from build123d import *

# Parameters (mm, degrees)
SKETCH_2_R      = 1.7
EXTRUDE_1_DEPTH = 3
EXTRUDE_2_DEPTH = 3.5
FILLET_5_R      = 1


with BuildPart() as part:
    # ｽｹｯﾁ2 → ﾎﾞｽ - 押し出し1 (new body)
    with BuildSketch(Plane(origin=(0, 0, 0), x_dir=(1, 0, 0), z_dir=(0, 1, 0))):
        with BuildLine():
            Line((85.95, 71.05), (89.45, 71.05))
            ThreePointArc((89.45, 71.05), (93.45, 67.05), (89.45, 63.05))
            Line((89.45, 63.05), (85.95, 63.05))
            Line((85.95, 63.05), (85.95, 8))
            Line((85.95, 8), (89.45, 8))
            ThreePointArc((89.45, 8), (93.45, 4), (89.45, 0))
            Line((89.45, 0), (85.95, 0))
            Line((85.95, 0), (0, 0))
            Line((0, 0), (-3.5, 0))
            ThreePointArc((-3.5, 0), (-7.5, 4), (-3.5, 8))
            Line((-3.5, 8), (0, 8))
            Line((0, 8), (0, 63.05))
            Line((0, 63.05), (-3.5, 63.05))
            ThreePointArc((-3.5, 63.05), (-7.5, 67.05), (-3.5, 71.05))
            Line((-3.5, 71.05), (0, 71.05))
            Line((0, 71.05), (85.95, 71.05))
        make_face()
        with Locations(Location((89.45, 67.05, 0), (0, 0, 270))):
            Circle(SKETCH_2_R, mode=Mode.SUBTRACT)
        with Locations(Location((89.45, 4, 0), (0, 0, 270))):
            Circle(SKETCH_2_R, mode=Mode.SUBTRACT)
        with Locations(Location((-3.5, 67.05, 0), (0, 0, 270))):
            Circle(SKETCH_2_R, mode=Mode.SUBTRACT)
        with Locations(Location((-3.5, 4, 0), (0, 0, 270))):
            Circle(SKETCH_2_R, mode=Mode.SUBTRACT)
    extrude(amount=EXTRUDE_1_DEPTH)

    # ｽｹｯﾁ3 → ﾎﾞｽ - 押し出し2 (add)
    with BuildSketch(Plane(origin=(0, 3, 0), x_dir=(1, 0, 0), z_dir=(0, 1, 0))):
        Polygon((68.9, 0), (70.5, 5.5), (70.5, 7.5), (67.5, 7.5), (67.5, 0), align=None)
        Polygon((67.5, 15.5), (70.5, 15.5), (70.5, 70.05), (82.95, 70.05), (82.95, 0), (85.95, 0), (85.95, 71.05), (67.5, 71.05), align=None)
        Polygon((45, 15.5), (48, 15.5), (48, 70.05), (60.45, 70.05), (60.45, 0), (63.45, 0), (63.45, 71.05), (45, 71.05), align=None)
        Polygon((46.4, 0), (48, 5.5), (48, 7.5), (45, 7.5), (45, 0), align=None)
        Polygon((22.5, 15.5), (25.5, 15.5), (25.5, 70.05), (37.95, 70.05), (37.95, 0), (40.95, 0), (40.95, 71.05), (22.5, 71.05), align=None)
        Polygon((23.9, 0), (25.5, 5.5), (25.5, 7.5), (22.5, 7.5), (22.5, 0), align=None)
        Polygon((0, 15.5), (3, 15.5), (3, 70.05), (15.45, 70.05), (15.45, 0), (18.45, 0), (18.45, 71.05), (0, 71.05), align=None)
        Polygon((1.4, 0), (3, 5.5), (3, 7.5), (0, 7.5), (0, 0), align=None)
    extrude(amount=EXTRUDE_2_DEPTH)

    # ﾌｨﾚｯﾄ5
    fillet_5_edges = [part.edges().sort_by_distance(p)[0] for p in [
        (85.95, 4.75, 0),
        (85.95, 4.75, -71.05),
        (45, 4.75, -71.05),
        (60.45, 4.75, 0),
        (63.45, 4.75, 0),
        (63.45, 4.75, -71.05),
        (22.5, 4.75, 0),
        (22.5, 4.75, -71.05),
        (37.95, 4.75, 0),
        (40.95, 4.75, 0),
        (40.95, 4.75, -71.05),
        (0, 4.75, 0),
        (0, 4.75, -71.05),
        (15.45, 4.75, 0),
        (18.45, 4.75, 0),
        (18.45, 4.75, -71.05),
        (67.5, 4.75, 0),
        (45, 4.75, 0),
        (67.5, 4.75, -71.05),
        (82.95, 4.75, 0),
    ]]
    fillet(fillet_5_edges, radius=FILLET_5_R)


solid = part.part
Design review of the part built by this model. Coordinates are the model's own, in mm. A direction names the side the tool comes from. Round coordinates to 2 decimals unless told otherwise and drop trailing zeros. Loops run counter-clockwise (first coordinate to the right, second up) from the corner with the lowest first, then second, coordinate; pieces in that order, holes last. Notation, with made-up numbers: (-35, 65.25) -> (-11, 65.25) arc R25 ccw to (-11, 88.25) -> close; hole circle Ø3 at (5, 71). An arc over 180 degrees is marked (long way). Use one line per item in the form item = value. Start each with the question number.
Q1. For pin 1 Ø6.5 at (x, z) = (90.5, -2.5) entering from +Y; pin 2 Ø1.5 at (x, z) = (26.5, -15) entering from -Y; pin 3 Ø2 at (y, z) = (4.5, -6.5) entering from +X; pin 4 Ø3 at (y, z) = (4.5, -22.5) entering from -X, all flat-tipped, find the tip position at first contact; note any pin that passes through.
Q2. Machinability: for faces 4 (the face through (3, 5, -42)), 5 (the face through (22.5, 5, -43)), 6 (the face through (-4.2, 1.5, -65.5)), 7 (the face through (69, 5, -15.5)), which of the approach directions +Z, -Z, +X, -X, +Y, -Y give a long, thin tool a straight path to every point of the face, cutting with its end or side? Answer none if there is none.
Q3. Wall thickness on line 1 along Z through (x, y) = (89.45, 1.55); line 2 along X through (y, z) = (1.7, -67.05); line 3 along X through (y, z) = (0.5, -65.5): over which ranges is each line inside the solid? List them lowest first. Write a range as [from, to].
Q4. We need section B-B on x = 53. Give the boundary of the cut face in (y, z).
Q5. We need section C-C on y = 4.75. State how many separate pieces and enclosed holes the cut face has, then the cut area to 3 significant figures.
Q6. Draft analysis for pull direction X (two halves, no side actions). For faces 1 (the face through (93.45, 1.48, -67.14)), 2 (the face through (22.5, 5, -4)), 3 (the face through (44, 2, 0)), state which applies: +X half, -X half, draft (parallel to the pull), parting line (faces both ways), or undercut.
Calculated:
q1.pin_1 = 3
q1.pin_2 = 0
q1.pin_3 = 85.95
q1.pin_4 = 0
q2.face_4 = +Z, +Y
q2.face_5 = +Z, -Z, +Y
q2.face_6 = +Y, -Y
q2.face_7 = +Y
q3.line_1 = [-71.05, -68.75], [-65.35, -63.05], [-8, -5.7], [-2.3, 0]
q3.line_2 = [-7.5, -5.2], [-1.8, 87.75], [91.15, 93.45]
q3.line_3 = [-7.19, -4.2], [-2.8, 88.75], [90.15, 93.14]
q4.outline = (0, -71.05) -> (6.5, -71.05) -> (6.5, -70.05) -> (3, -70.05) -> (3, 0) -> (0, 0) -> close
q5.separate_pieces = 8
q5.enclosed_holes = 0
q5.area = 1,640 mm²
q6.face_1 = +X half
q6.face_2 = undercut
q6.face_3 = draft
